from build123d import *

# Parameters (mm, degrees)
SKETCH1_W                                        = 25.4
SKETCH1_H                                        = 25.4
BOSS_EXTRUDE1_DEPTH                              = 7
CBORE_FOR_1_4_SOCKET_HEAD_CAP_SCREW1_D           = 6.7564
CBORE_FOR_1_4_SOCKET_HEAD_CAP_SCREW1_CBORE_D     = 11.1125
CBORE_FOR_1_4_SOCKET_HEAD_CAP_SCREW1_CBORE_DEPTH = 6.35
SKETCH4_W                                        = 7.14375
SKETCH4_H                                        = 12.7
BOSS_EXTRUDE2_DEPTH                              = 25.4
SKETCH5_W                                        = 7.14375
SKETCH5_H                                        = 3
BOSS_EXTRUDE3_DEPTH                              = 25.4
FILLET1_R                                        = 10
FILLET2_START                                    = -14
FILLET2_DEPTH                                    = 28
FILLET2_START_2                                  = -12.7
FILLET2_2_DEPTH                                  = 12.604348727
FILLET2_START_3                                  = 7
FILLET2_3_DEPTH                                  = 10.0000001


with BuildPart() as part:
    # Sketch1 → Boss-Extrude1 (new body)
    with BuildSketch(Plane.XY):
        Rectangle(SKETCH1_W, SKETCH1_H)
    extrude(amount=BOSS_EXTRUDE1_DEPTH)

    # CBORE for 1/4 Socket Head Cap Screw1 (through all)
    with Locations(Plane.XY.offset(7)):
        with Locations((0, 0)):
            CounterBoreHole(CBORE_FOR_1_4_SOCKET_HEAD_CAP_SCREW1_D / 2, CBORE_FOR_1_4_SOCKET_HEAD_CAP_SCREW1_CBORE_D / 2, CBORE_FOR_1_4_SOCKET_HEAD_CAP_SCREW1_CBORE_DEPTH)

    # Sketch4 → Boss-Extrude2 (add)
    with BuildSketch(Plane.XY.offset(7)):
        with Locations((-9.128125, -6.35)):
            Rectangle(SKETCH4_W, SKETCH4_H)
        with Locations((9.128125, -6.35)):
            Rectangle(SKETCH4_W, SKETCH4_H)
    extrude(amount=BOSS_EXTRUDE2_DEPTH)

    # Sketch5 → Boss-Extrude3 (add)
    with BuildSketch(Plane(origin=(0, 0, 0), x_dir=(1, 0, 0), z_dir=(0, 1, 0))):
        with Locations((-9.128125, -30.9)):
            Rectangle(SKETCH5_W, SKETCH5_H)
        with Locations((9.128125, -30.9)):
            Rectangle(SKETCH5_W, SKETCH5_H)
    extrude(amount=BOSS_EXTRUDE3_DEPTH)

    # Fillet1
    # the kernel refuses this fillet: 10 mm, written as the material it adds along each edge
    with BuildSketch(Plane(origin=(-19.44375, 0, 7), x_dir=(0, 1, 0), z_dir=(1, 0, 0))) as fillet1_piece_1_section:
        with BuildLine():
            CenterArc((FILLET1_R, FILLET1_R), FILLET1_R, 180, 90)
            Line((0, FILLET1_R), (0, 0))
            Line((0, 0), (FILLET1_R, 0))
        make_face()
    fillet1_piece_1 = extrude(amount=32.14375, mode=Mode.PRIVATE)
    fillet1_piece_1 = fillet1_piece_1 - Plane(origin=(0, 0, 7), x_dir=(1, 0, 0), z_dir=(0, 0, 1)) * Cylinder(5.55625, 105, mode=Mode.PRIVATE)
    fillet1_piece_1 = split(fillet1_piece_1, bisect_by=Plane(origin=(-12.7, 0, 7), z_dir=(1, 0, 0)), keep=Keep.TOP, mode=Mode.PRIVATE)
    add(fillet1_piece_1)
    with BuildSketch(Plane(origin=(-12.7, 0, 29.4), x_dir=(0, 0, -1), z_dir=(1, 0, 0))) as fillet1_piece_2:
        with BuildLine():
            CenterArc((FILLET1_R, FILLET1_R), FILLET1_R, 180, 90)
            Line((0, FILLET1_R), (0, 0))
            Line((0, 0), (FILLET1_R, 0))
        make_face()
    extrude(amount=7.14375)
    with BuildSketch(Plane(origin=(-37.7, 0, 29.4), x_dir=(0, 0, -1), z_dir=(1, 0, 0))) as fillet1_piece_3_section:
        with BuildLine():
            CenterArc((FILLET1_R, FILLET1_R), FILLET1_R, 180, 90)
            Line((0, FILLET1_R), (0, 0))
            Line((0, 0), (FILLET1_R, 0))
        make_face()
    fillet1_piece_3 = extrude(amount=57.14375, mode=Mode.PRIVATE)
    fillet1_piece_3 = split(fillet1_piece_3, bisect_by=Plane(origin=(5.55625, 0, 29.4), z_dir=(1, 0, 0)), keep=Keep.TOP, mode=Mode.PRIVATE)
    fillet1_piece_3 = split(fillet1_piece_3, bisect_by=Plane(origin=(12.7, 0, 29.4), z_dir=(-1, 0, 0)), keep=Keep.TOP, mode=Mode.PRIVATE)
    add(fillet1_piece_3)
    with BuildSketch(Plane(origin=(12.7, 0, 29.4), x_dir=(0, 0, -1), z_dir=(-1, 0, 0))) as fillet1_piece_4:
        with BuildLine():
            CenterArc((FILLET1_R, -FILLET1_R), FILLET1_R, 90, 90)
            Line((0, -FILLET1_R), (0, 0))
            Line((0, 0), (FILLET1_R, 0))
        make_face()
    extrude(amount=7.14375)
    with BuildSketch(Plane(origin=(37.7, 0, 29.4), x_dir=(0, 0, -1), z_dir=(-1, 0, 0))) as fillet1_piece_5_section:
        with BuildLine():
            CenterArc((FILLET1_R, -FILLET1_R), FILLET1_R, 90, 90)
            Line((0, -FILLET1_R), (0, 0))
            Line((0, 0), (FILLET1_R, 0))
        make_face()
    fillet1_piece_5 = extrude(amount=57.14375, mode=Mode.PRIVATE)
    fillet1_piece_5 = split(fillet1_piece_5, bisect_by=Plane(origin=(-12.7, 0, 29.4), z_dir=(1, 0, 0)), keep=Keep.TOP, mode=Mode.PRIVATE)
    fillet1_piece_5 = split(fillet1_piece_5, bisect_by=Plane(origin=(-5.55625, 0, 29.4), z_dir=(-1, 0, 0)), keep=Keep.TOP, mode=Mode.PRIVATE)
    add(fillet1_piece_5)
    # the kernel refuses this fillet: 10 mm, written as the material it takes off along each edge
    with BuildSketch(Plane(origin=(-37.7, -12.7, 32.4), x_dir=(0, 0, -1), z_dir=(1, 0, 0))) as fillet1_2_piece_1:
        with BuildLine():
            CenterArc((FILLET1_R, FILLET1_R), FILLET1_R, 180, 90)
            Line((0, FILLET1_R), (0, 0))
            Line((0, 0), (FILLET1_R, 0))
        make_face()
    extrude(amount=57.14375, mode=Mode.SUBTRACT)
    with BuildSketch(Plane(origin=(37.7, -12.7, 32.4), x_dir=(0, 0, -1), z_dir=(-1, 0, 0))) as fillet1_2_piece_2:
        with BuildLine():
            CenterArc((FILLET1_R, -FILLET1_R), FILLET1_R, 90, 90)
            Line((0, -FILLET1_R), (0, 0))
            Line((0, 0), (FILLET1_R, 0))
        make_face()
    extrude(amount=57.14375, mode=Mode.SUBTRACT)

    # Fillet2: read off the stored shape, not the designer's step
    # Fillet2 outline → Fillet2 (cut)
    with BuildSketch(Plane.YZ.offset(FILLET2_START)):
        with BuildLine():
            ThreePointArc((10, 7), (9.231056683, 7.029607521), (8.466666667, 7.118254765))
            ThreePointArc((8.466666667, 7.118254765), (11.496928583, 5.430585697), (12.7, 2.177382148))
            Line((12.7, 2.177382148), (12.7, 7))
            Line((12.7, 7), (10, 7))
        make_face()
        with BuildLine():
            Line((25.4, 29.4), (25.4, 32.4))
            ThreePointArc((25.4, 32.4), (23.556037093, 30.216699867), (20.817424305, 29.4))
            Line((20.817424305, 29.4), (25.4, 29.4))
        make_face()
    extrude(amount=FILLET2_DEPTH, mode=Mode.SUBTRACT)

    # Fillet2 2 outline → Fillet2 2 (add)
    with BuildSketch(Plane(origin=(0, 0, 0), x_dir=(1, 0, 0), z_dir=(0, 1, 0)).offset(FILLET2_START_2)):
        with BuildLine():
            Line((5.55625, -7), (0.55625, -7))
            ThreePointArc((0.55625, -7), (4.091783906, -8.464466094), (5.55625, -12))
            Line((5.55625, -12), (5.55625, -7))
        make_face()
        with BuildLine():
            ThreePointArc((-5.55625, -12), (-4.091783906, -8.464466094), (-0.55625, -7))
            Line((-0.55625, -7), (-5.55625, -7))
            Line((-5.55625, -7), (-5.55625, -12))
        make_face()
    extrude(amount=FILLET2_2_DEPTH)

    # Fillet2 3 outline → Fillet2 3 (cut)
    with BuildSketch(Plane.XY.offset(FILLET2_START_3)):
        with BuildLine():
            ThreePointArc((5.555426617, -0.095651273), (0, 5.55625), (-5.555426617, -0.095651273))
            ThreePointArc((-5.555426617, -0.095651273), (0, -5.55625), (5.555426617, -0.095651273))
        make_face()
    extrude(amount=FILLET2_3_DEPTH, mode=Mode.SUBTRACT)


solid = part.part
Work out the finished part from the listing and answer in its coordinate system (mm). A direction names the side the tool comes from. Give positions to 0.01 mm unless a question says otherwise; leave off trailing zeros. Order: outer loops, then holes, each group sorted by start corner. A loop starts at its lowest first (then second) coordinate and runs counter-clockwise, first axis right, second up. Notation, with made-up numbers: (41.25, 8) -> (72.25, 8) arc R18 ccw to (72.25, 24) -> close; hole circle Ø4 at (47, -4). An arc over 180 degrees is marked (long way). One line per item, written item: value.
Item 1: Find section C-C, the plane x = 10.25. Give the vertices of the cut face in (y, z), plus the area to 3 significant figures.
Answer sheet:
outline: (-12.7, 0) -> (12.7, 0) -> (12.7, 2.18) arc R5 ccw to (8.47, 7.12) arc R10 cw to (0, 17) -> (0, 19.4) arc R10 cw to (10, 29.4) -> (20.82, 29.4) arc R5 ccw to (25.4, 32.4) -> (-2.7, 32.4) arc R10 ccw to (-12.7, 22.4) -> close
area: 590 mm²
Item 2: Find section A-A, the plane z = 23. Give the vertices of the cut face in (x, y).
Answer sheet:
outline: (-12.7, -12.68) -> (-5.56, -12.68) -> (-5.56, 0.67) -> (-12.7, 0.67) -> close; (5.56, -12.68) -> (12.7, -12.68) -> (12.7, 0.67) -> (5.56, 0.67) -> close
Item 3: Determine the mould class of faces 6 (the flat face through (-12.7, -2, 16)), 7 (the cylindrical face through (-9.18, 3.01, 26.55)), 8 (the flat face through (5.556, -2, 24)) for opening direction X: released by +X, released by -X, zero draft, split by the parting line, or undercut.
Answer sheet:
face 6: released by -X
face 7: zero draft
face 8: undercut
Item 4: Flat-ended cylindrical pins translate along their axes: P1, Ø0.6, axis at x = 0, y = -8, coming from the +Z side; P2, Ø12, axis at y = 17.5, z = 11, coming from the +X side; P3, Ø3.5, axis at x = -8, y = 14.5, coming from the -Z side; P4, Ø5, axis at x = -1.5, z = 8.5, coming from the -Y side. Find the tip coordinate at first contact, or state that the pin passes through.
Answer sheet:
P1: z = 7
P2: through
P3: z = 29.4
P4: y = -12.7
Item 5: A tool of negligible diameter and unlimited length cuts with its end or side. For faces 1 (the flat face through (0, -12.7, 6)), 2 (the flat face through (9, 12, 32.4)), 3 (the cylindrical face through (-4.7, -7.9, 9.2)), 4 (the flat face through (9, 0, 18)), 5 (the flat face through (0, -4, 0.65)), from which of +Z, -Z, +X, -X, +Y, -Y can it reach the whole face along a straight path? Write none if from no direction.
Answer sheet:
face 1: +Z, -Z, +X, -X, -Y
face 2: +Z, +X, -X, +Y, -Y
face 3: +Z, -Y
face 4: +X, -X, +Y
face 5: +Z
Item 6: Find section B-B, the plane y = 5. Give the vertices of the cut face in (x, z), plus the area to 3 significant figures.
Answer sheet:
outline: (-12.7, 0) -> (12.7, 0) -> (12.7, 8.34) -> (2.42, 8.34) -> (2.42, 0.65) -> (-2.42, 0.65) -> (-2.42, 8.34) -> (-12.7, 8.34) -> close; (-12.7, 28.06) -> (-5.56, 28.06) -> (-5.56, 32.4) -> (-12.7, 32.4) -> close; (5.56, 28.06) -> (12.7, 28.06) -> (12.7, 32.4) -> (5.56, 32.4) -> close
area: 237 mm²
Item 7: Straight lines are drawn through the part: probe 1 along X at (y, z) = (0, 4); probe 2 along Y at (x, z) = (0, 0.55). For each, find the intervals that lie inside material, in ascending order.
Answer sheet:
probe 1: -12.7 to -5.56, 5.56 to 12.7
probe 2: -12.7 to -3.38, 3.38 to 12.7
Item 8: Find section D-D, the plane x = 0. Give the vertices of the cut face in (y, z), plus the area to 3 significant figures.
Answer sheet:
outline: (-12.7, 0) -> (-3.38, 0) -> (-3.38, 0.65) -> (-5.56, 0.65) -> (-5.56, 7) -> (-12.7, 7) -> close; (3.38, 0) -> (12.7, 0) -> (12.7, 2.18) arc R5 ccw to (8.47, 7.12) arc R10 cw to (5.56, 8.04) -> (5.56, 0.65) -> (3.38, 0.65) -> close
area: 99.7 mm²
